```python
from build123d import *

# Parameters (mm, degrees)
SKETCH1_R           = 3.25
BOSS_EXTRUDE1_DEPTH = 12.5
SKETCH2_R           = 1.75
CUT_EXTRUDE1_DEPTH  = 2.5
SKETCH6_R           = 4.8
BOSS_EXTRUDE2_DEPTH = 5
BOSS_EXTRUDE3_DEPTH = 1
FILLET1_R           = 0.75


with BuildPart() as part:
    # Sketch1 → Boss-Extrude1 (new body)
    with BuildSketch(Plane(origin=(0, 0, 0), x_dir=(1, 0, 0), z_dir=(0, 1, 0))):
        Circle(SKETCH1_R)
    extrude(amount=BOSS_EXTRUDE1_DEPTH)

    # Sketch2 → Cut-Extrude1 (cut)
    with BuildSketch(Plane.XZ):
        Circle(SKETCH2_R)
    extrude(amount=-CUT_EXTRUDE1_DEPTH, mode=Mode.SUBTRACT)

    # Sketch6 → Boss-Extrude2 (add)
    with BuildSketch(Plane(origin=(0, 12.5, 0), x_dir=(1, 0, 0), z_dir=(0, 1, 0))):
        Circle(SKETCH6_R)
    extrude(amount=BOSS_EXTRUDE2_DEPTH)

    # Sketch12 → Boss-Extrude3 (add)
    with BuildSketch(Plane(origin=(0, 17.5, 0), x_dir=(1, 0, 0), z_dir=(0, 1, 0))):
        Polygon((0, 3.542487974), (-2.95, 0.842487974), (-2.25, 0.842487974), (-2.25, -3.157512026), (-0.9, -3.172366953), (-0.9, -0.972366953), (0.9, -0.972366953), (0.9, -3.172366953), (2.25, -3.157512026), (2.25, 0.842487974), (2.95, 0.842487974), align=None)
    extrude(amount=BOSS_EXTRUDE3_DEPTH)

    # Fillet1
    fillet1_edges = [part.edges().sort_by_distance(p)[0] for p in [
        (-4.8, 17.5, 0),
    ]]
    fillet(fillet1_edges, radius=FILLET1_R)


solid = part.part
```
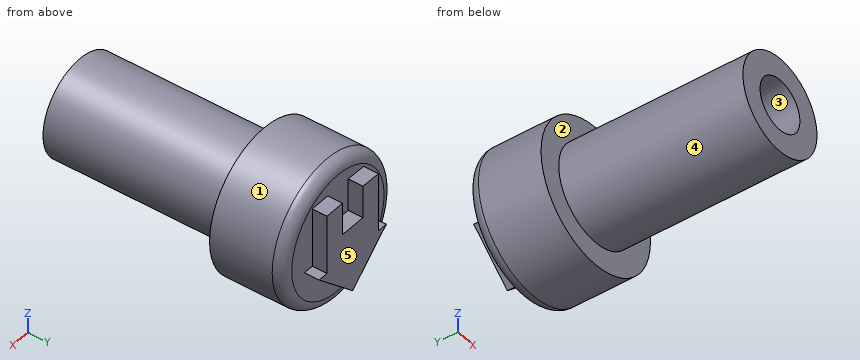
Geometry: final body of the model. Coordinates: model frame, mm. Face numbers are marked on the shaded views. A direction names the side the tool comes from. Coordinates: 2 decimals unless noted, no trailing zeros. Order: outer loops, then holes, each group sorted by start corner. A loop starts at its lowest first (then second) coordinate and runs counter-clockwise, first axis right, second up. Notation, with made-up numbers: (23, -22) -> (63, -22) arc R23 ccw to (63, -2) -> close; hole circle Ø1 at (-28.5, 37). An arc over 180 degrees is marked (long way). Write each question's results on one line, items separated by ' | '. Start each with the question number.
1) Cut plane D-D, the plane y = 8.25. Output: boundary loops of the cut face in (x, z), and give its area (3 significant figures).
2) Set-up query: the marked faces 4 and 5. Return all of +Z, -Z, +X, -X, +Y, -Y with unobstructed straight access to the full face (end or side cutting, diameter ignored); none if empty.
3) Cut plane C-C, the plane y = 14. Output: boundary loops of the cut face in (x, z), and give its area (3 significant figures).
4) Cut plane B-B, the plane z = 0. Output: boundary loops of the cut face in (x, y), and give its area (3 significant figures).
5) Cut plane A-A, the plane y = 2.25. Output: boundary loops of the cut face in (x, z).
6) Mould query, pull axis X, two halves, no side actions, for the marked faces 1, 2 and 3. Classes: released by +X, released by -X, zero draft, split by the parting line, or undercut.
7) Material intervals for line 1 along Z through (x, y) = (0, 1.3); line 2 along Y through (x, z) = (4, 1); line 3 along Y through (x, z) = (-1, -2.75), sorted ascending.
8) First-contact query: pin 1 (4 mm diameter, centred on y = 7, z = 2, fed in from -X); pin 2 (0.8 mm diameter, centred on y = 18, z = 1.5, fed in from +X); pin 3 (0.8 mm diameter, centred on x = 3, y = 18, fed in from +Z); pin 4 (5 mm diameter, centred on x = -2, y = 11, fed in from +Z). Flat tips, straight axial feed; report the tip coordinate or a pass-through.
Checks:
1) outline: circle Ø6.5 at (0, 0) | area: 33.2 mm^2
2) face 4: -Y | face 5: +Z, -Z, +X, -X, +Y
3) outline: circle Ø9.6 at (0, 0) | area: 72.4 mm^2
4) outline: (-4.8, 12.5) -> (-3.25, 12.5) -> (-3.25, 0) -> (-1.75, 0) -> (-1.75, 2.5) -> (1.75, 2.5) -> (1.75, 0) -> (3.25, 0) -> (3.25, 12.5) -> (4.8, 12.5) -> (4.8, 16.75) arc R0.75 ccw to (4.05, 17.5) -> (2.25, 17.5) -> (2.25, 18.5) -> (-2.25, 18.5) -> (-2.25, 17.5) -> (-4.05, 17.5) arc R0.75 ccw to (-4.8, 16.75) -> close | area: 125 mm^2
5) outline: circle Ø6.5 at (0, 0); hole circle Ø3.5 at (0, 0)
6) face 1: split by the parting line | face 2: zero draft | face 3: undercut
7) line 1: -3.25 to -1.75, 1.75 to 3.25 | line 2: 12.5 to 17.5 | line 3: 0 to 17.5
8) pin 1: x = -3.25 | pin 2: x = 2.25 | pin 3: z = -0.84 | pin 4: z = 4.8
